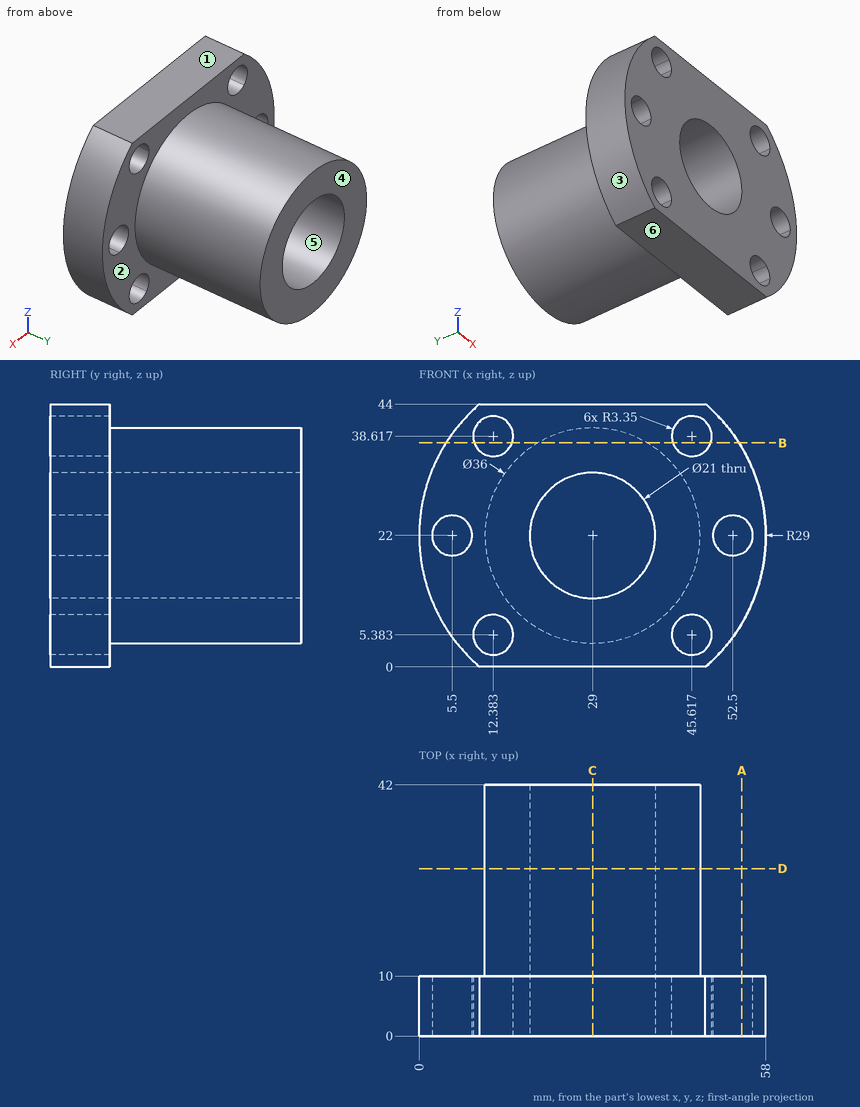
Answer from the drawing. Dimensions are ordinates in mm from the lowest x, y and z of the part. A direction names the side the tool comes from. Round coordinates to 2 decimals unless told otherwise and drop trailing zeros. Write each loop counter-clockwise with the first axis right and the second up, starting at its lowest first coordinate (ties: lowest second). Pieces come first, ordered by that corner, then holes. Notation, with made-up numbers: M 75,-33.5 L 133,-33.5 A15 ccw 133,-23.5 Z; hole C 71.25,42.25 d9. An arc over 180 degrees is marked long. Write each question's results on one line, items separated by ' | '. Start each with the question number.
Item 1: Find section A-A on x = 54. Write down the section's boundary in (y, z).
Item 2: Find section D-D on y = 28. Write down the section's boundary in (x, z).
Item 3: Given pin 1 Ø8 at (x, y) = (32.5, 26.5) entering from +Z; pin 2 Ø1 at (x, y) = (31, 23.5) entering from -Z; pin 3 Ø10 at (y, z) = (34.5, 17.5) entering from -X; pin 4 Ø17 at (x, z) = (29, 22) entering from -Y, each flat-ended and moving along its own axis, determine where each tip first touches the part or whether it passes through.
Item 4: Find section C-C on x = 29. Write down the section's boundary in (y, z).
Item 5: The mould has two halves that part along Z. Classify the marked faces 3, 4, 5 and 6: +Z half, -Z half, draft (parallel to the pull), parting line (faces both ways), or undercut.
Item 6: Which of the six approach directions +Z, -Z, +X, -X, +Y, -Y give full straight-line access (tool end or side, diameter ignored) to the marked faces 1 and 2?
Item 7: Find section B-B on z = 37.5. Write down the section's boundary in (x, y), and give its area (3 significant figures).
Item 8: Straight lines are drawn through the part: probe 1 along Z at (x, y) = (29, 14); probe 2 along Z at (x, y) = (28.5, 2); probe 3 along X at (y, z) = (7.5, 38). For each, find the intervals that lie inside material, in ascending order.
Answer block:
1) outline: M 0,7.3 L 10,7.3 L 10,19 L 0,19 Z; M 0,25 L 10,25 L 10,36.7 L 0,36.7 Z
2) outline: C 29,22 d36; hole C 29,22 d21
3) pin 1: stops at z = 40 | pin 2: stops at z = 4.06 | pin 3: stops at x = 11 | pin 4: passes through
4) outline: M 0,0 L 10,0 L 10,4 L 42,4 L 42,11.5 L 0,11.5 Z; M 0,32.5 L 42,32.5 L 42,40 L 10,40 L 10,44 L 0,44 Z
5) face 3: parting line | face 4: draft | face 5: undercut | face 6: -Z half
6) face 1: +Z, +X, -X, +Y, -Y | face 2: +Y
7) outline: M 4.49,0 L 9.22,0 L 9.22,10 L 4.49,10 Z; M 15.54,0 L 42.46,0 L 42.46,10 L 38.15,10 L 38.15,42 L 19.85,42 L 19.85,10 L 15.54,10 Z; M 48.78,0 L 53.51,0 L 53.51,10 L 48.78,10 Z | area: 950 mm²
8) probe 1: z = 4 to 11.5, 32.5 to 40 | probe 2: z = 0 to 11.51, 32.49 to 44 | probe 3: x = 4.81 to 9.09, 15.68 to 42.32, 48.91 to 53.19
